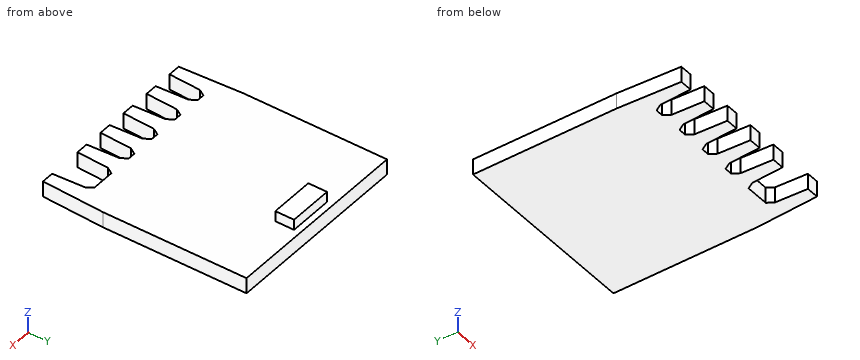
from build123d import *

# Parameters (mm, degrees)
BOSS_EXTRUDE1_DEPTH = 1.5
BOSS_EXTRUDE3_START = 1.5
SKETCH11_W          = 4.3
SKETCH11_H          = 1.8
BOSS_EXTRUDE3_DEPTH = 1


with BuildPart() as part:
    # Sketch1 → Boss-Extrude1 (new body)
    with BuildSketch(Plane.XY):
        Polygon((0, 6), (0.314446676, 0), (1.497941481, 0), (1.657221927, 3.039251967), (2.042586863, 3.65596478), (2.769801294, 3.65596478), (3.155166229, 3.039251967), (3.314446676, 0), (4.497941481, 0), (4.657221927, 3.039251967), (5.042586863, 3.65596478), (5.769801294, 3.65596478), (6.155166229, 3.039251967), (6.314446676, 0), (7.497941481, 0), (7.657221927, 3.039251967), (8.042586863, 3.65596478), (8.769801294, 3.65596478), (9.155166229, 3.039251967), (9.314446676, 0), (10.497941481, 0), (10.657221927, 3.039251967), (11.042586863, 3.65596478), (11.769801294, 3.65596478), (12.155166229, 3.039251967), (12.314446676, 0), (13.497941481, 0), (13.657221927, 3.039251967), (14.042586863, 3.65596478), (16.269801294, 3.65596478), (16.655166229, 3.039251967), (16.814446676, 0), (17.997941481, 0), (18.312388157, 6), (18.312388157, 19.8), (0, 19.8), align=None)
    extrude(amount=BOSS_EXTRUDE1_DEPTH)

    # Sketch11 → Boss-Extrude3 (add)
    with BuildSketch(Plane.XY.offset(BOSS_EXTRUDE3_START)):
        with Locations((9.156194078, 18.3)):
            Rectangle(SKETCH11_W, SKETCH11_H)
    extrude(amount=BOSS_EXTRUDE3_DEPTH)


solid = part.part
Input: part model. Units: mm. Frame: model coordinates. Round coordinates to 2 decimals unless told otherwise and drop trailing zeros. Loops run counter-clockwise (first coordinate to the right, second up) from the corner with the lowest first, then second, coordinate; pieces in that order, holes last. Notation, with made-up numbers: (49.25, -10) -> (65.25, -10) arc R20 cw to (65.25, 29) -> close; hole circle Ø8 at (-20, 23.25). An arc over 180 degrees is marked (long way). Answer as a JSON object with one key per item and string values. Group by question number.
1) Pin query (flat end, axial travel): pin 1 (6 mm diameter, centred on x = 8, y = 15.5, fed in from -Z); pin 2 (1.5 mm diameter, centred on x = 14.5, y = 11.5, fed in from +Z); pin 3 (0.8 mm diameter, centred on x = 8.5, z = 0.5, fed in from -Y); pin 4 (0.5 mm diameter, centred on x = 9.5, z = 2, fed in from -Y). Return the tip coordinate at first contact, or that it passes through.
2) Section query B-B on z = 1.8. Output: boundary loops of the cut face in (x, y).
3) Section query A-A on x = 17.25. Output: boundary loops of the cut face in (y, z), plus the area to 3 significant figures.
4) Ray query, L1, parallel to X at y = 1.75, z = 0.6; L2, parallel to Z at x = 12.25, y = 10.5; L3, parallel to Y at x = 5.25, z = 1.05. Return the intervals inside material, ascending.
Reply:
{
 "1": {"pin 1": "stops at z = 0", "pin 2": "stops at z = 1.5", "pin 3": "stops at y = 3.45", "pin 4": "stops at y = 17.4"},
 "2": {"outline": "(7.01, 17.4) -> (11.31, 17.4) -> (11.31, 19.2) -> (7.01, 19.2) -> close"},
 "3": {"outline": "(0, 0) -> (19.8, 0) -> (19.8, 1.5) -> (0, 1.5) -> close", "area": "29.7 mm2"},
 "4": {"L1": "x = 0.22 to 1.59, 3.22 to 4.59, 6.22 to 7.59, 9.22 to 10.59, 12.22 to 13.59, 16.72 to 18.09", "L2": "z = 0 to 1.5", "L3": "y = 3.66 to 19.8"}
}
